```python
from build123d import *

# Parameters (mm, degrees)
EXTRUDE_1_DEPTH     = 10
SKETCH_4_W          = 5
SKETCH_4_H          = 8
EXTRUDE_3_DEPTH     = 3
EXTRUDE_4_DEPTH     = 16
CUT_EXTRUDE_1_DEPTH = 11
SKETCH_15_W         = 5
SKETCH_15_H         = 20
EXTRUDE_5_DEPTH     = 22
OTHER_START         = -1
OTHER_4_OUTLINE_R   = 1.6
OTHER_4_DEPTH       = 32


# Read off the part's stored shape, not the designer's step: 高级异型孔3, 高级异型孔4
with BuildPart() as part:
    # 草图1 → 凸台-拉伸1 (new body)
    with BuildSketch(Plane(origin=(0, 0, 0), x_dir=(1, 0, 0), z_dir=(0, 1, 0))):
        Polygon((0, 10), (0, 30), (30, 30), (30, 10), (31, 0), (30, 0), (0, 0), (-1, 0), align=None)
    extrude(amount=-EXTRUDE_1_DEPTH)

    # 草图4 → 凸台-拉伸3 (add)
    with BuildSketch(Plane(origin=(0, 0, 0), x_dir=(1, 0, 0), z_dir=(0, 1, 0))):
        with Locations((2.5, 15)):
            Rectangle(SKETCH_4_W, SKETCH_4_H)
        with Locations((27.5, 15)):
            Rectangle(SKETCH_4_W, SKETCH_4_H)
    extrude(amount=EXTRUDE_3_DEPTH)

    # 高级异型孔3 outline → 高级异型孔3 (revolve, cut)
    with BuildSketch(Plane(origin=(15, 0, -15), x_dir=(1, 0, 0), z_dir=(0, 0, 1))):
        Polygon((0, -10), (3.15, -10), (1.7, -8.55), (1.7, 0), (0, 0), align=None)
    revolve(axis=Axis((15, 0, -15), (0, 1, 0)), mode=Mode.SUBTRACT)

    # 草图13 → 凸台-拉伸4 (add, symmetric)
    with BuildSketch(Plane(origin=(15, 0, 0), x_dir=(0, 0, -1), z_dir=(1, 0, 0))):
        with BuildLine():
            Line((0, -10), (0, 15))
            Line((0, 15), (0, 72))
            ThreePointArc((0, 72), (-10, 82), (-20, 72))
            Line((-20, 72), (-20, 10.908419296))
            Line((-20, 10.908419296), (-20, 0.454209648))
            Line((-20, 0.454209648), (-10, -10))
            Line((-10, -10), (0, -10))
        make_face()
    extrude(amount=EXTRUDE_4_DEPTH, both=True)

    # 草图13<2> → 切除-拉伸1 (cut, symmetric)
    with BuildSketch(Plane(origin=(15, 0, 0), x_dir=(0, 0, -1), z_dir=(1, 0, 0))):
        with BuildLine():
            Line((0, -10), (0, 15))
            Line((0, 15), (0, 72))
            ThreePointArc((0, 72), (-10, 82), (-20, 72))
            Line((-20, 72), (-20, 10.908419296))
            Line((-20, 10.908419296), (-20, 0.454209648))
            Line((-20, 0.454209648), (-10, -10))
            Line((-10, -10), (0, -10))
        make_face()
    extrude(amount=CUT_EXTRUDE_1_DEPTH, both=True, mode=Mode.SUBTRACT)

    # 草图15 → 凸台-拉伸5 (add)
    with BuildSketch(Plane(origin=(4, 0, 0), x_dir=(0, 0, -1), z_dir=(1, 0, 0))):
        with Locations((-10, 47)):
            Rectangle(SKETCH_15_W, SKETCH_15_H)
    extrude(amount=EXTRUDE_5_DEPTH)

    # 高级异型孔4 outline → 高级异型孔4 (cut)
    with BuildSketch(Plane.YZ.offset(OTHER_START)):
        with Locations((72, 10)):
            Circle(OTHER_4_OUTLINE_R)
    extrude(amount=OTHER_4_DEPTH, mode=Mode.SUBTRACT)


solid = part.part
```
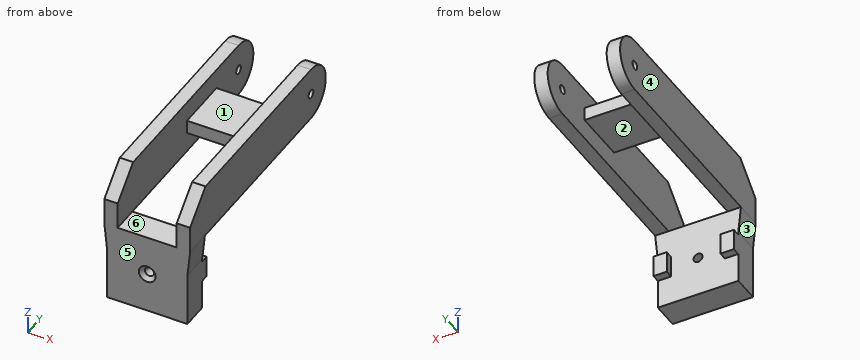
Work out the finished part from the listing and answer in its coordinate system (mm). Face numbers are marked on the shaded views. A direction names the side the tool comes from. Round coordinates to 2 decimals unless told otherwise and drop trailing zeros. Loops run counter-clockwise (first coordinate to the right, second up) from the corner with the lowest first, then second, coordinate; pieces in that order, holes last.
(1) The part is cut by section D-D, the plane x = 23. Give the vertices of the cut face in (y, z).
Computed values:
outline: (-10, -30) - (0, -30) - (0, 0) - (-10, 0) - close; (37, 7.5) - (57, 7.5) - (57, 12.5) - (37, 12.5) - close
(2) The part is cut by section C-C, the plane x = 2.5. Give the vertices of the cut face in (y, z).
Computed values:
outline: (-10, -30) - (0, -30) - (0, -19) - (3, -19) - (3, -11) - (0, -11) - (0, 0) - (72, 0) arc R10 ccw to (72, 20) - (0.45, 20) - (-10, 10) - close; hole circle Ø3.2 at (72, 10)
(3) The mould has two halves that part along X. Classify the marked faces 4, 5 and 6: pulls with the +X half, pulls with the -X half, needs draft (parallel to the pull), parting line crosses it, or undercut.
Computed values:
face 4: pulls with the -X half
face 5: needs draft
face 6: undercut
(4) For the marked faces 1, 2 and 3, determine the directions among +Z, -Z, +X, -X, +Y, -Y from which every point of the face is accessible in a straight line to the end or side of a thin tool.
Computed values:
face 1: +Z, +Y, -Y
face 2: -Z, +Y, -Y
face 3: -Z, -X, +Y, -Y
(5) Each of these flat-tipped pins is pushed along its axis until it touches: P1, Ø2.5, axis at x = 16, z = 10.5, coming from the -Y side; P2, Ø1.5, axis at y = 1.5, z = -13.5, coming from the -X side; P3, Ø6, axis at x = 11.5, y = 43, coming from the -Z side; P4, Ø5, axis at y = 7.5, z = -1.5, coming from the -X side. Where does it stop, or does it pass through?
Computed values:
P1: stops at y = 37
P2: stops at x = 0
P3: stops at z = 7.5
P4: stops at x = -1
(6) Find the intervals of material crossed by L1, parallel to Z at x = 1.85, y = 72; L2, parallel to Y at x = 29, z = 10; L3, parallel to X at y = 0.5, z = -17.5, in increasing order.
Computed values:
L1: z = 0 to 8.4, 11.6 to 20
L2: y = -10 to 70.4, 73.6 to 82
L3: x = 0 to 5, 25 to 30
(7) The part is cut by section B-B, the plane y = 6. Give the vertices of the cut face in (x, z).
Computed values:
outline: (-1, 0) - (4, 0) - (4, 20) - (-1, 20) - close; (26, 0) - (31, 0) - (31, 20) - (26, 20) - close
(8) The part is cut by section A-A, the plane z = -15. Give the vertices of the cut face in (x, y), and give its area (3 significant figures).
Computed values:
outline: (0, -10) - (11.85, -10) - (13.3, -8.55) - (13.3, 0) - (5, 0) - (5, 3) - (0, 3) - close; (16.7, -8.55) - (18.15, -10) - (30, -10) - (30, 3) - (25, 3) - (25, 0) - (16.7, 0) - close
area: 294 mm2
